from build123d import *

# Parameters (mm, degrees)
BOSS_EXTRUDE1_DEPTH = 3
FILLET1_R           = 200
FILLET2_R           = 10
CUT_EXTRUDE2_DEPTH  = 429.345808882
SKETCH3_W           = 42
SKETCH3_H           = 23
SKETCH3_H_2         = 19
CUT_EXTRUDE3_DEPTH  = 429.345808882
SKETCH4_R           = 1.6
CUT_EXTRUDE5_DEPTH  = 429.345808882
SKETCH5_R           = 1.6
CUT_EXTRUDE6_DEPTH  = 429.345808882
SKETCH6_W           = 66
SKETCH6_H           = 15
SKETCH6_R           = 1.6
BOSS_EXTRUDE2_DEPTH = 3
FILLET3_R           = 5
SKETCH7_R           = 1.6
CUT_EXTRUDE7_DEPTH  = 435.224748243
SKETCH9_R           = 1.6
CUT_EXTRUDE8_DEPTH  = 435.224748243
SKETCH10_W          = 302
SKETCH10_H          = 255.8
CUT_EXTRUDE9_DEPTH  = 10
BOSS_EXTRUDE5_DEPTH = 3
CUT_EXTRUDE10_DEPTH = 10


with BuildPart() as part:
    # Sketch1 → Boss-Extrude1 (new body)
    with BuildSketch(Plane(origin=(0, 0, 0), x_dir=(1, 0, 0), z_dir=(0, 1, 0))):
        Polygon((0, 0), (170, 0), (170, 300), (225, 300), (225, 367.51288694), (85, 330), (-55, 367.51288694), (-55, 300), (0, 300), align=None)
    extrude(amount=BOSS_EXTRUDE1_DEPTH)

    # Fillet1
    fillet1_edges = [part.edges().sort_by_distance(p)[0] for p in [
        (85, 1.5, -330),
    ]]
    fillet(fillet1_edges, radius=FILLET1_R)

    # Fillet2
    fillet2_edges = [part.edges().sort_by_distance(p)[0] for p in [
        (0, 1.5, -300),
        (-55, 1.5, -300),
        (-55, 1.5, -367.51288694),
        (225, 1.5, -367.51288694),
        (225, 1.5, -300),
        (170, 1.5, -300),
        (170, 1.5, 0),
        (0, 1.5, 0),
    ]]
    fillet(fillet2_edges, radius=FILLET2_R)

    # Sketch2 → Cut-Extrude2 (cut, through all)
    with BuildSketch(Plane(origin=(0, 3, 0), x_dir=(1, 0, 0), z_dir=(0, 1, 0))):
        with BuildLine():
            ThreePointArc((132.5, 80), (118.587572106, 113.587572106), (85, 127.5))
            Line((85, 127.5), (85, 32.5))
            ThreePointArc((85, 32.5), (118.587572106, 46.412427894), (132.5, 80))
        make_face()
        with BuildLine():
            Line((85, 32.5), (85, 127.5))
            ThreePointArc((85, 127.5), (37.5, 80), (85, 32.5))
        make_face()
    extrude(amount=-CUT_EXTRUDE2_DEPTH, mode=Mode.SUBTRACT)

    # Sketch3 → Cut-Extrude3 (cut, through all)
    with BuildSketch(Plane(origin=(0, 3, 0), x_dir=(1, 0, 0), z_dir=(0, 1, 0))):
        with Locations((40, 267.3)):
            Rectangle(SKETCH3_W, SKETCH3_H)
        with Locations((130, 267.3)):
            Rectangle(SKETCH3_W, SKETCH3_H)
        with Locations((40, 9.5)):
            Rectangle(SKETCH3_W, SKETCH3_H_2)
        with Locations((130, 9.5)):
            Rectangle(SKETCH3_W, SKETCH3_H_2)
    extrude(amount=-CUT_EXTRUDE3_DEPTH, mode=Mode.SUBTRACT)

    # Sketch4 → Cut-Extrude5 (cut, through all)
    with BuildSketch(Plane(origin=(0, 3, 0), x_dir=(1, 0, 0), z_dir=(0, 1, 0))):
        with Locations(Location((85, 133, 0), (0, 0, 270))):
            Circle(SKETCH4_R)
        with Locations(Location((122.476659403, 117.476659403, 0), (0, 0, 270))):
            Circle(SKETCH4_R)
        with Locations(Location((138, 80, 0), (0, 0, 270))):
            Circle(SKETCH4_R)
        with Locations(Location((122.476659403, 42.523340597, 0), (0, 0, 270))):
            Circle(SKETCH4_R)
        with Locations(Location((85, 27, 0), (0, 0, 270))):
            Circle(SKETCH4_R)
        with Locations(Location((47.523340597, 42.523340597, 0), (0, 0, 270))):
            Circle(SKETCH4_R)
        with Locations(Location((32, 80, 0), (0, 0, 270))):
            Circle(SKETCH4_R)
        with Locations(Location((47.523340597, 117.476659403, 0), (0, 0, 270))):
            Circle(SKETCH4_R)
    extrude(amount=-CUT_EXTRUDE5_DEPTH, mode=Mode.SUBTRACT)

    # Sketch5 → Cut-Extrude6 (cut, through all)
    with BuildSketch(Plane(origin=(0, 3, 0), x_dir=(1, 0, 0), z_dir=(0, 1, 0))):
        with Locations(Location((7.5, 312, 0), (0, 0, 270))):
            Circle(SKETCH5_R)
        with Locations(Location((7.5, 267.3, 0), (0, 0, 270))):
            Circle(SKETCH5_R)
        with Locations(Location((7.5, 222.3, 0), (0, 0, 270))):
            Circle(SKETCH5_R)
        with Locations(Location((7.5, 97.5, 0), (0, 0, 270))):
            Circle(SKETCH5_R)
        with Locations(Location((7.5, 7.5, 0), (0, 0, 270))):
            Circle(SKETCH5_R)
        with Locations(Location((7.5, 52.5, 0), (0, 0, 270))):
            Circle(SKETCH5_R)
        with Locations(Location((70, 7.5, 0), (0, 0, 270))):
            Circle(SKETCH5_R)
        with Locations(Location((100, 7.5, 0), (0, 0, 270))):
            Circle(SKETCH5_R)
        with Locations(Location((162.5, 7.5, 0), (0, 0, 270))):
            Circle(SKETCH5_R)
        with Locations(Location((162.5, 52.5, 0), (0, 0, 270))):
            Circle(SKETCH5_R)
        with Locations(Location((162.5, 97.5, 0), (0, 0, 270))):
            Circle(SKETCH5_R)
        with Locations(Location((162.5, 222.3, 0), (0, 0, 270))):
            Circle(SKETCH5_R)
        with Locations(Location((162.5, 267.3, 0), (0, 0, 270))):
            Circle(SKETCH5_R)
        with Locations(Location((162.5, 312, 0), (0, 0, 270))):
            Circle(SKETCH5_R)
        with Locations(Location((162.5, 342.75495241, 0), (0, 0, 270))):
            Circle(SKETCH5_R)
        with Locations(Location((109.337835254, 328.510193298, 0), (0, 0, 270))):
            Circle(SKETCH5_R)
        with Locations(Location((60.662164746, 328.510193298, 0), (0, 0, 270))):
            Circle(SKETCH5_R)
        with Locations(Location((7.5, 342.75495241, 0), (0, 0, 270))):
            Circle(SKETCH5_R)
        with Locations(Location((70, 267.5, 0), (0, 0, 270))):
            Circle(SKETCH5_R)
        with Locations(Location((100, 267.5, 0), (0, 0, 270))):
            Circle(SKETCH5_R)
    extrude(amount=-CUT_EXTRUDE6_DEPTH, mode=Mode.SUBTRACT)

    # Sketch6 → Boss-Extrude2 (add)
    # profile 1 of 2: a face of its own
    with BuildSketch(Plane.XZ):
        with Locations((-33, -52.5)):
            Rectangle(SKETCH6_W, SKETCH6_H)
        with Locations(Location((-45, -52.5, 0), (0, 0, 270))):
            Circle(SKETCH6_R, mode=Mode.SUBTRACT)
        with Locations(Location((-21, -52.5, 0), (0, 0, 270))):
            Circle(SKETCH6_R, mode=Mode.SUBTRACT)
    # profile 2 of 2: a face of its own
    with BuildSketch(Plane.XZ):
        with Locations((203, -52.5)):
            Rectangle(SKETCH6_W, SKETCH6_H)
        with Locations(Location((191, -52.5, 0), (0, 0, 270))):
            Circle(SKETCH6_R, mode=Mode.SUBTRACT)
        with Locations(Location((215, -52.5, 0), (0, 0, 270))):
            Circle(SKETCH6_R, mode=Mode.SUBTRACT)
    extrude(amount=-BOSS_EXTRUDE2_DEPTH)

    # Fillet3
    fillet3_edges = [part.edges().sort_by_distance(p)[0] for p in [
        (19, 1.5, 0),
        (61, 1.5, 0),
        (109, 1.5, 0),
        (109, 1.5, -19),
        (151, 1.5, -19),
        (151, 1.5, 0),
        (0, 1.5, -45),
        (0, 1.5, -60),
        (-66, 1.5, -60),
        (-66, 1.5, -45),
        (170, 1.5, -60),
        (170, 1.5, -45),
        (236, 1.5, -45),
        (236, 1.5, -60),
    ]]
    fillet(fillet3_edges, radius=FILLET3_R)

    # Sketch7 → Cut-Extrude7 (cut, through all)
    with BuildSketch(Plane(origin=(0, 3, 0), x_dir=(1, 0, 0), z_dir=(0, 1, 0))):
        with Locations(Location((130, 171.5, 0), (0, 0, 270))):
            Circle(SKETCH7_R)
        with Locations(Location((145, 171.5, 0), (0, 0, 270))):
            Circle(SKETCH7_R)
        with Locations(Location((145, 159.5, 0), (0, 0, 270))):
            Circle(SKETCH7_R)
        with Locations(Location((130, 159.5, 0), (0, 0, 270))):
            Circle(SKETCH7_R)
        with Locations(Location((25, 171.5, 0), (0, 0, 270))):
            Circle(SKETCH7_R)
        with Locations(Location((40, 171.5, 0), (0, 0, 270))):
            Circle(SKETCH7_R)
        with Locations(Location((40, 159.5, 0), (0, 0, 270))):
            Circle(SKETCH7_R)
        with Locations(Location((25, 159.5, 0), (0, 0, 270))):
            Circle(SKETCH7_R)
        with Locations(Location((70, 242, 0), (0, 0, 270))):
            Circle(SKETCH7_R)
        with Locations(Location((100, 242, 0), (0, 0, 270))):
            Circle(SKETCH7_R)
    extrude(amount=-CUT_EXTRUDE7_DEPTH, mode=Mode.SUBTRACT)

    # Sketch9 → Cut-Extrude8 (cut, through all)
    with BuildSketch(Plane(origin=(0, 3, 0), x_dir=(1, 0, 0), z_dir=(0, 1, 0))):
        with Locations(Location((-45, 307.5, 0), (0, 0, 270))):
            Circle(SKETCH9_R)
        with Locations(Location((-15, 307.5, 0), (0, 0, 270))):
            Circle(SKETCH9_R)
        with Locations(Location((-45, 327.5, 0), (0, 0, 270))):
            Circle(SKETCH9_R)
        with Locations(Location((-15, 327.5, 0), (0, 0, 270))):
            Circle(SKETCH9_R)
        with Locations(Location((185, 307.5, 0), (0, 0, 90))):
            Circle(SKETCH9_R)
        with Locations(Location((185, 327.5, 0), (0, 0, 90))):
            Circle(SKETCH9_R)
        with Locations(Location((215, 307.5, 0), (0, 0, 90))):
            Circle(SKETCH9_R)
        with Locations(Location((215, 327.5, 0), (0, 0, 90))):
            Circle(SKETCH9_R)
    extrude(amount=-CUT_EXTRUDE8_DEPTH, mode=Mode.SUBTRACT)

    # Sketch10 → Cut-Extrude9 (cut)
    with BuildSketch(Plane(origin=(0, 3, 0), x_dir=(1, 0, 0), z_dir=(0, 1, 0))):
        with Locations((85, 127.9)):
            Rectangle(SKETCH10_W, SKETCH10_H)
    extrude(amount=-CUT_EXTRUDE9_DEPTH, mode=Mode.SUBTRACT)

    # Sketch11 → Boss-Extrude5 (add)
    with BuildSketch(Plane(origin=(0, 3, 0), x_dir=(1, 0, 0), z_dir=(0, 1, 0))):
        with BuildLine():
            Line((33.236190979, 343.870070824), (12.5, 349.426316451))
            Line((12.5, 349.426316451), (157.5, 349.426316451))
            Line((157.5, 349.426316451), (136.763809021, 343.870070824))
            ThreePointArc((136.763809021, 343.870070824), (85, 337.055236082), (33.236190979, 343.870070824))
        make_face()
    extrude(amount=-BOSS_EXTRUDE5_DEPTH)

    # Sketch12 → Cut-Extrude10 (cut)
    with BuildSketch(Plane(origin=(0, 3, 0), x_dir=(1, 0, 0), z_dir=(0, 1, 0))):
        with BuildLine():
            Line((50.9, 341.426316451), (50.9, 291.426316451))
            ThreePointArc((50.9, 291.426316451), (52.5, 289.826316451), (54.1, 291.426316451))
            Line((54.1, 291.426316451), (54.1, 341.426316451))
            ThreePointArc((54.1, 341.426316451), (52.5, 343.026316451), (50.9, 341.426316451))
        make_face()
        with BuildLine():
            Line((83.4, 341.426316451), (83.4, 291.426316451))
            ThreePointArc((83.4, 291.426316451), (85, 289.826316451), (86.6, 291.426316451))
            Line((86.6, 291.426316451), (86.6, 341.426316451))
            ThreePointArc((86.6, 341.426316451), (85, 343.026316451), (83.4, 341.426316451))
        make_face()
        with BuildLine():
            Line((115.9, 341.426316451), (115.9, 291.426316451))
            ThreePointArc((115.9, 291.426316451), (117.5, 289.826316451), (119.1, 291.426316451))
            Line((119.1, 291.426316451), (119.1, 341.426316451))
            ThreePointArc((119.1, 341.426316451), (117.5, 343.026316451), (115.9, 341.426316451))
        make_face()
    extrude(amount=-CUT_EXTRUDE10_DEPTH, mode=Mode.SUBTRACT)


solid = part.part
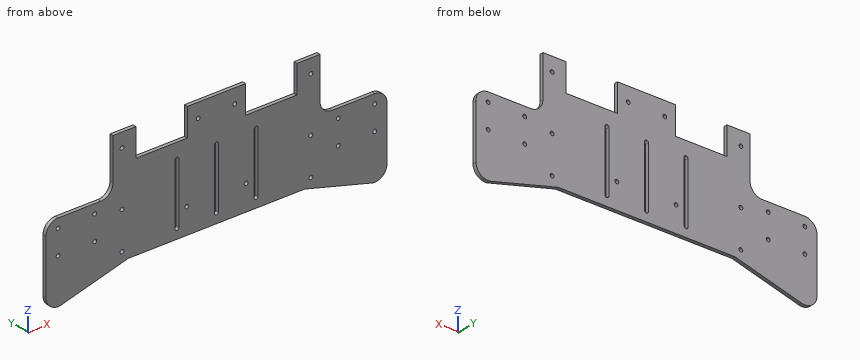
The listing builds one solid part. Answer for the finished solid, in the listing's coordinates (mm). Coordinates: 2 decimals unless noted, no trailing zeros. Order: outer loops, then holes, each group sorted by start corner. A loop starts at its lowest first (then second) coordinate and runs counter-clockwise, first axis right, second up. Notation, with made-up numbers: (3, 8) -> (35, 8) arc R29 cw to (35, 34) -> close; hole circle Ø2 at (-32.75, -13). An arc over 180 degrees is marked (long way). Answer in a Markdown table with one row per item. Add a question column.
Item 1: Find section C-C (y = 1). State how many separate pieces and enclosed holes the cut face has, then the cut area to 3 significant figures.
Item 2: Find the intervals of material crossed by L1, parallel to X at y = 1, z = -333.5; L2, parallel to X at y = 2.2, z = -271; L3, parallel to Z at x = 185, y = 1.9, in increasing order. Write a range as from..to.
Item 3: Find section D-D (x = 177). Write down the section's boundary in (y, z), then the cut area to 3 significant figures.
Item 4: Find section B-B (x = 31.5). Write down the section's boundary in (y, z), then the cut area to 3 significant figures.
Item 5: Each of these flat-tipped pins is pushed along its axis until it touches: P1, Ø0.9, axis at x = 120.5, y = 1.5, coming from the +Z side; P2, Ø3, axis at x = 70, z = -267.5, coming from the -Y side; P3, Ø1.5, axis at y = 1.5, z = -266, coming from the -X side; P4, Ø5, axis at x = 162.5, z = -312, coming from the +Y side. Where does it stop, or does it pass through?
Item 6: Find section A-A (z = -320.5). Write down the section's boundary in (x, y), then the cut area to 3 significant figures.
Result set:
| question | item | result |
|---|---|---|
| 1 | separate pieces | 1 |
| 1 | enclosed holes | 21 |
| 1 | area | 19,900 mm² |
| 2 | L1 | x = -55..50.9, 54.1..83.4, 86.6..115.9, 119.1..225 |
| 2 | L2 | x = 0..19, 61..109, 151..170 |
| 2 | L3 | z = -356.79..-329.1, -325.9..-309.1, -305.9..-300 |
| 3 | outline | (0, -354.65) -> (3, -354.65) -> (3, -299.54) -> (0, -299.54) -> close |
| 3 | area | 165 mm² |
| 4 | outline | (0, -349.43) -> (3, -349.43) -> (3, -278.8) -> (0, -278.8) -> close |
| 4 | area | 212 mm² |
| 5 | P1 | stops at z = -278.8 |
| 5 | P2 | passes through |
| 5 | P3 | stops at x = 0 |
| 5 | P4 | stops at y = 3 |
| 6 | outline | (-55, 0) -> (50.9, 0) -> (50.9, 3) -> (-55, 3) -> close; (54.1, 0) -> (83.4, 0) -> (83.4, 3) -> (54.1, 3) -> close; (86.6, 0) -> (115.9, 0) -> (115.9, 3) -> (86.6, 3) -> close; (119.1, 0) -> (225, 0) -> (225, 3) -> (119.1, 3) -> close |
| 6 | area | 811 mm² |
